Read the model definition and answer for the solid it produces. Units are mm, in the model's axes. Give positions to 0.01 mm unless a question says otherwise; leave off trailing zeros. Order: outer loops, then holes, each group sorted by start corner. A loop starts at its lowest first (then second) coordinate and runs counter-clockwise, first axis right, second up. Notation, with made-up numbers: (-26.5, 15.25) - (-21.5, 15.25) arc R19 cw to (-21.5, 51.25) - close; hole circle Ø5 at (43, -1). An arc over 180 degrees is marked (long way). Write each question's results on one line, items separated by ' | '. Start each with the question number.
Q1. Find section B-B on y = -1.75. Count the separate pieces of the cut face and the enclosed holes in it, and give its area (3 significant figures).
Q2. Find section A-A on x = -30. Give the vertices of the cut face in (y, z).
Q3. Find section C-C on z = 16. Give the vertices of the cut face in (x, y).
Q4. Flat-ended cylindrical pins translate along their axes: P1, Ø10, axis at x = -44.45, z = 50.47, coming from the -Y side; P2, Ø1, axis at x = -48, y = -4.5, coming from the +Z side; P3, Ø2, axis at x = -25.5, y = -3.5, coming from the -Z side; P4, Ø3, axis at x = -10.5, y = -3.5, coming from the -Z side. Find the tip coordinate at first contact, or state that the pin passes through.
Q5. Find the intervals of material crossed by line 1 along Z through (x, y) = (-44.45, -3.25); line 2 along Z through (x, y) = (0, -4.25); line 3 along Z through (x, y) = (-49, -6), in increasing order. Write a range as from..to.
Q6. Find section D-D on x = -38.5. Give the vertices of the cut face in (y, z) (3 decimals).
from build123d import *

# Parameters (mm, degrees)
F0_R        = 3.175
F0_R_2      = 1.5875
F1_DEPTH    = 3.048
F1_FACE_R   = 3.175
F1_FACE_R_2 = 1.5875
F2_DEPTH    = 3.048


# Not quite as in the source:
# - after a boolean that leaves OpenCascade's solid faulty, fix() repairs it


with BuildPart() as f1:
    # F0 (on Front) → F1 (new body)
    with BuildSketch(Plane.XZ):
        with BuildLine():
            ThreePointArc((-53.975, 50.4670464277), (-44.45, 40.9420464277), (-34.925, 50.4670464277))
            ThreePointArc((-34.925, 50.4670464277), (-44.45, 59.9920464277), (-53.975, 50.4670464277))
        make_face()
        with Locations((-44.45, 50.4670464277)):
            Circle(F0_R, mode=Mode.SUBTRACT)
        with BuildLine():
            Line((-28.7025430953, 1.6753357581), (-34.925, 50.4670464277))
            ThreePointArc((-34.925, 50.4670464277), (-44.45, 40.9420464277), (-53.975, 50.4670464277))
            Line((-53.975, 50.4670464277), (-59.4731707335, 4.7973452602))
            ThreePointArc((-59.4731707335, 4.7973452602), (-42.8475383164, 15.4609611278), (-28.7025430953, 1.6753357581))
        make_face()
        with Locations((-48.45572263, 36.1922464277)):
            Circle(F0_R_2, mode=Mode.SUBTRACT)
        with BuildLine():
            ThreePointArc((-28.575, -0.3329535723), (-28.6069178604, 0.6732140673), (-28.7025430953, 1.6753357581))
            ThreePointArc((-28.7025430953, 1.6753357581), (-42.8475383164, 15.4609611278), (-59.4731707335, 4.7973452602))
            ThreePointArc((-59.4731707335, 4.7973452602), (-60.0824637934, 2.4314090575), (-60.3215080228, 0))
            Line((-60.3215080228, 0), (-59.9501789354, -3.7622505804))
            ThreePointArc((-59.9501789354, -3.7622505804), (-43.7288188136, -16.1915639369), (-28.7025430953, -2.3412429026))
            ThreePointArc((-28.7025430953, -2.3412429026), (-28.6069178604, -1.3391212118), (-28.575, -0.3329535723))
        make_face()
        with Locations((-44.45, -0.3329535723)):
            Circle(F0_R, mode=Mode.SUBTRACT)
        with BuildLine():
            Line((-59.9501789354, -3.7622505804), (-60.3215080228, 0))
            ThreePointArc((-60.3215080228, 0), (-60.2482378134, -1.8922184603), (-59.9501789354, -3.7622505804))
        make_face()
        with BuildLine():
            Line((-33.1183182382, -46.317436026), (-28.7025430953, -2.3412429026))
            ThreePointArc((-28.7025430953, -2.3412429026), (-43.7288188136, -16.1915639369), (-59.9501789354, -3.7622505804))
            Line((-59.9501789354, -3.7622505804), (-53.928942688, -64.7685125051))
            ThreePointArc((-53.928942688, -64.7685125051), (-44.9183459706, -54.3194748683), (-34.925, -63.8329535723))
            ThreePointArc((-34.925, -63.8329535723), (-37.4756032752, -70.3201267105), (-43.7614126668, -73.3330310711))
            Line((-43.7614126668, -73.3330310711), (0.2823318858, -71.7654307992))
            ThreePointArc((0.2823318858, -71.7654307992), (-7.9374918809, -63.8443065466), (0.2596391732, -55.8997011655))
            Line((0.2596391732, -55.8997011655), (-25.4679521782, -55.0576895661))
            ThreePointArc((-25.4679521782, -55.0576895661), (-31.1901358295, -52.3480122444), (-33.1183182382, -46.317436026))
        make_face()
        with BuildLine():
            ThreePointArc((-34.925, -63.8329535723), (-44.9183459706, -54.3194748683), (-53.928942688, -64.7685125051))
            ThreePointArc((-53.928942688, -64.7685125051), (-50.8501155234, -70.8873242945), (-44.4614490432, -73.3579466914))
            Line((-44.4614490432, -73.3579466914), (-43.7614126668, -73.3330310711))
            ThreePointArc((-43.7614126668, -73.3330310711), (-37.4756032752, -70.3201267105), (-34.925, -63.8329535723))
        make_face()
        with Locations((-44.45, -63.8329535723)):
            Circle(F0_R, mode=Mode.SUBTRACT)
        with BuildLine():
            Line((-43.7614126668, -73.3330310711), (-44.4614490432, -73.3579466914))
            ThreePointArc((-44.4614490432, -73.3579466914), (-44.111201737, -73.3519262446), (-43.7614126668, -73.3330310711))
        make_face()
        with BuildLine():
            ThreePointArc((7.9375, -63.8329535723), (5.7037177432, -58.3128530156), (0.2596391732, -55.8997011655))
            ThreePointArc((0.2596391732, -55.8997011655), (-7.9374918809, -63.8443065466), (0.2823318858, -71.7654307992))
            ThreePointArc((0.2823318858, -71.7654307992), (5.7116072866, -69.344890478), (7.9375, -63.8329535723))
        make_face()
        with Locations((0, -63.8329535723)):
            Circle(F0_R, mode=Mode.SUBTRACT)
    extrude(amount=F1_DEPTH)

    # F0 (on Front) + F1_face (on face) → F2 (join)
    with BuildSketch(Plane.XZ):
        with BuildLine():
            ThreePointArc((-53.975, 50.4670464277), (-44.45, 40.9420464277), (-34.925, 50.4670464277))
            ThreePointArc((-34.925, 50.4670464277), (-44.45, 59.9920464277), (-53.975, 50.4670464277))
        make_face()
        with Locations((-44.45, 50.4670464277)):
            Circle(F0_R, mode=Mode.SUBTRACT)
        with BuildLine():
            Line((-28.7025430953, 1.6753357581), (-34.925, 50.4670464277))
            ThreePointArc((-34.925, 50.4670464277), (-44.45, 40.9420464277), (-53.975, 50.4670464277))
            Line((-53.975, 50.4670464277), (-59.4731707335, 4.7973452602))
            ThreePointArc((-59.4731707335, 4.7973452602), (-42.8475383164, 15.4609611278), (-28.7025430953, 1.6753357581))
        make_face()
        with Locations((-48.45572263, 36.1922464277)):
            Circle(F0_R_2, mode=Mode.SUBTRACT)
        with BuildLine():
            ThreePointArc((-28.575, -0.3329535723), (-28.6069178604, 0.6732140673), (-28.7025430953, 1.6753357581))
            ThreePointArc((-28.7025430953, 1.6753357581), (-42.8475383164, 15.4609611278), (-59.4731707335, 4.7973452602))
            ThreePointArc((-59.4731707335, 4.7973452602), (-60.0824637934, 2.4314090575), (-60.3215080228, 0))
            Line((-60.3215080228, 0), (-59.9501789354, -3.7622505804))
            ThreePointArc((-59.9501789354, -3.7622505804), (-43.7288188136, -16.1915639369), (-28.7025430953, -2.3412429026))
            ThreePointArc((-28.7025430953, -2.3412429026), (-28.6069178604, -1.3391212118), (-28.575, -0.3329535723))
        make_face()
        with Locations((-44.45, -0.3329535723)):
            Circle(F0_R, mode=Mode.SUBTRACT)
        with BuildLine():
            Line((-59.9501789354, -3.7622505804), (-60.3215080228, 0))
            ThreePointArc((-60.3215080228, 0), (-60.2482378134, -1.8922184603), (-59.9501789354, -3.7622505804))
        make_face()
        with BuildLine():
            Line((-33.1183182382, -46.317436026), (-28.7025430953, -2.3412429026))
            ThreePointArc((-28.7025430953, -2.3412429026), (-43.7288188136, -16.1915639369), (-59.9501789354, -3.7622505804))
            Line((-59.9501789354, -3.7622505804), (-53.928942688, -64.7685125051))
            ThreePointArc((-53.928942688, -64.7685125051), (-44.9183459706, -54.3194748683), (-34.925, -63.8329535723))
            ThreePointArc((-34.925, -63.8329535723), (-37.4756032752, -70.3201267105), (-43.7614126668, -73.3330310711))
            Line((-43.7614126668, -73.3330310711), (0.2823318858, -71.7654307992))
            ThreePointArc((0.2823318858, -71.7654307992), (-7.9374918809, -63.8443065466), (0.2596391732, -55.8997011655))
            Line((0.2596391732, -55.8997011655), (-25.4679521782, -55.0576895661))
            ThreePointArc((-25.4679521782, -55.0576895661), (-31.1901358295, -52.3480122444), (-33.1183182382, -46.317436026))
        make_face()
        with BuildLine():
            ThreePointArc((-34.925, -63.8329535723), (-44.9183459706, -54.3194748683), (-53.928942688, -64.7685125051))
            ThreePointArc((-53.928942688, -64.7685125051), (-50.8501155234, -70.8873242945), (-44.4614490432, -73.3579466914))
            Line((-44.4614490432, -73.3579466914), (-43.7614126668, -73.3330310711))
            ThreePointArc((-43.7614126668, -73.3330310711), (-37.4756032752, -70.3201267105), (-34.925, -63.8329535723))
        make_face()
        with Locations((-44.45, -63.8329535723)):
            Circle(F0_R, mode=Mode.SUBTRACT)
        with BuildLine():
            Line((-43.7614126668, -73.3330310711), (-44.4614490432, -73.3579466914))
            ThreePointArc((-44.4614490432, -73.3579466914), (-44.111201737, -73.3519262446), (-43.7614126668, -73.3330310711))
        make_face()
        with BuildLine():
            ThreePointArc((7.9375, -63.8329535723), (5.7037177432, -58.3128530156), (0.2596391732, -55.8997011655))
            ThreePointArc((0.2596391732, -55.8997011655), (-7.9374918809, -63.8443065466), (0.2823318858, -71.7654307992))
            ThreePointArc((0.2823318858, -71.7654307992), (5.7116072866, -69.344890478), (7.9375, -63.8329535723))
        make_face()
        with Locations((0, -63.8329535723)):
            Circle(F0_R, mode=Mode.SUBTRACT)
    with BuildSketch(Plane(origin=(-39.2541813262, -3.048, -16.9379503901), x_dir=(1, 0, 0), z_dir=(0, -1, 0))):
        with BuildLine():
            ThreePointArc((4.3291813262, 67.4049968178), (-5.1958186738, 76.9299968178), (-14.7208186738, 67.4049968178))
            Line((-14.7208186738, 67.4049968178), (-20.2189894074, 21.7352956503))
            ThreePointArc((-20.2189894074, 21.7352956503), (-21.0462252614, 17.4883065075), (-20.6959976093, 13.1756998097))
            Line((-20.6959976093, 13.1756998097), (-14.6747613619, -47.830562115))
            ThreePointArc((-14.6747613619, -47.830562115), (-11.3322126787, -54.1799392572), (-4.5072313406, -56.395080681))
            Line((-4.5072313406, -56.395080681), (39.536513212, -54.8274804091))
            ThreePointArc((39.536513212, -54.8274804091), (47.1916732071, -46.8836502078), (39.5138204994, -38.9617507754))
            Line((39.5138204994, -38.9617507754), (13.7862291479, -38.119739176))
            ThreePointArc((13.7862291479, -38.119739176), (8.0640454966, -35.4100618543), (6.1358630879, -29.3794856359))
            Line((6.1358630879, -29.3794856359), (10.5516382309, 14.5967074875))
            ThreePointArc((10.5516382309, 14.5967074875), (10.6791813262, 16.6049968178), (10.5516382309, 18.6132861482))
            Line((10.5516382309, 18.6132861482), (4.3291813262, 67.4049968178))
        make_face()
        with Locations((-5.1958186738, 67.4049968178)):
            Circle(F1_FACE_R, mode=Mode.SUBTRACT)
        with Locations((-9.2015413039, 53.1301968178)):
            Circle(F1_FACE_R_2, mode=Mode.SUBTRACT)
        with Locations((-5.1958186738, 16.6049968178)):
            Circle(F1_FACE_R, mode=Mode.SUBTRACT)
        with Locations((-5.1958186738, -46.8950031822)):
            Circle(F1_FACE_R, mode=Mode.SUBTRACT)
        with Locations((39.2541813262, -46.8950031822)):
            Circle(F1_FACE_R, mode=Mode.SUBTRACT)
    extrude(amount=F2_DEPTH)

    add(f1.part.fix(), mode=Mode.REPLACE)


solid = f1.part
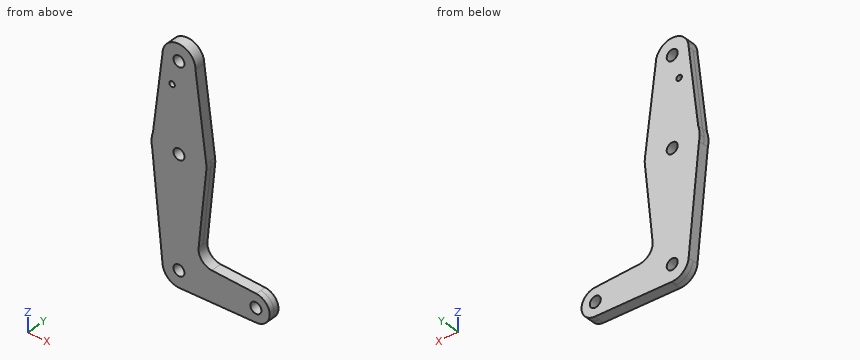
Working result:
1) separate pieces: 1 | enclosed holes: 5 | area: 3,780 mm²
2) outline: (-6.1, -72.84) - (0, -72.84) - (0, -53.46) - (-6.1, -53.46) - close; (-6.1, -15.26) - (0, -15.26) - (0, 11.85) - (-6.1, 11.85) - close
3) outline: (-58.12, -6.1) - (-30.53, -6.1) - (-30.53, 0) - (-58.12, 0) - close
4) P1: y = -6.1 | P2: z = 59.49 | P3: z = -72.72 | P4: z = -72.2
5) line 1: -73.36..-67.01, -60.66..-3.51, 2.84..47.29, 53.64..59.99 | line 2: -71.78..-67.01, -60.66..-55.89 | line 3: -72.2..34.7, 37.68..58.84
6) outline: (-6.096, -73.146) - (0, -73.146) - (0, 57.905) - (-6.096, 57.905) - close
